Can you work these out from the drawing? Everything is in mm from the part's minimum corner. A direction names the side the tool comes from. Give positions to 0.01 mm unless a question says otherwise; leave off trailing zeros. Order: outer loops, then holes, each group sorted by start corner. A loop starts at its lowest first (then second) coordinate and runs counter-clockwise, first axis right, second up. Notation, with made-up numbers: M -30.5,-11.75 L -2.5,-11.75 A15 ccw -2.5,0.25 Z; hole C 42.25,6.5 d9. An arc over 180 degrees is marked long. Use a Markdown table: item, result. Add a question column.
Item 1: For the marked faces 1, 2 and 3, which set-ups out of +Z, -Z, +X, -X, +Y, -Y let a thin tool reach every point of the face, with its end or its side?
Item 2: I'm going to push flat-ended pins straight in: pin 1 Ø1 at (x, y) = (132, 4.5) entering from -Z; pin 2 Ø1 at (x, y) = (46, 5.5) entering from +Z; pin 3 Ø8 at (x, z) = (49.5, 20) entering from +Y (1 decimal). Where does each tip first touch, or does it pass through?
Item 3: Suppose I cut it at A-A on y = 4.5. Write out the boundary of the cut face in (x, z) (1 decimal).
Item 4: If I drill on L1, parallel to Y at x = 115.5, z = 83.5 (1 decimal); L2, parallel to Z at x = 42, y = 4.75, over which ranges is the centre line in solid material (lowest first)? Write a range as from..to.
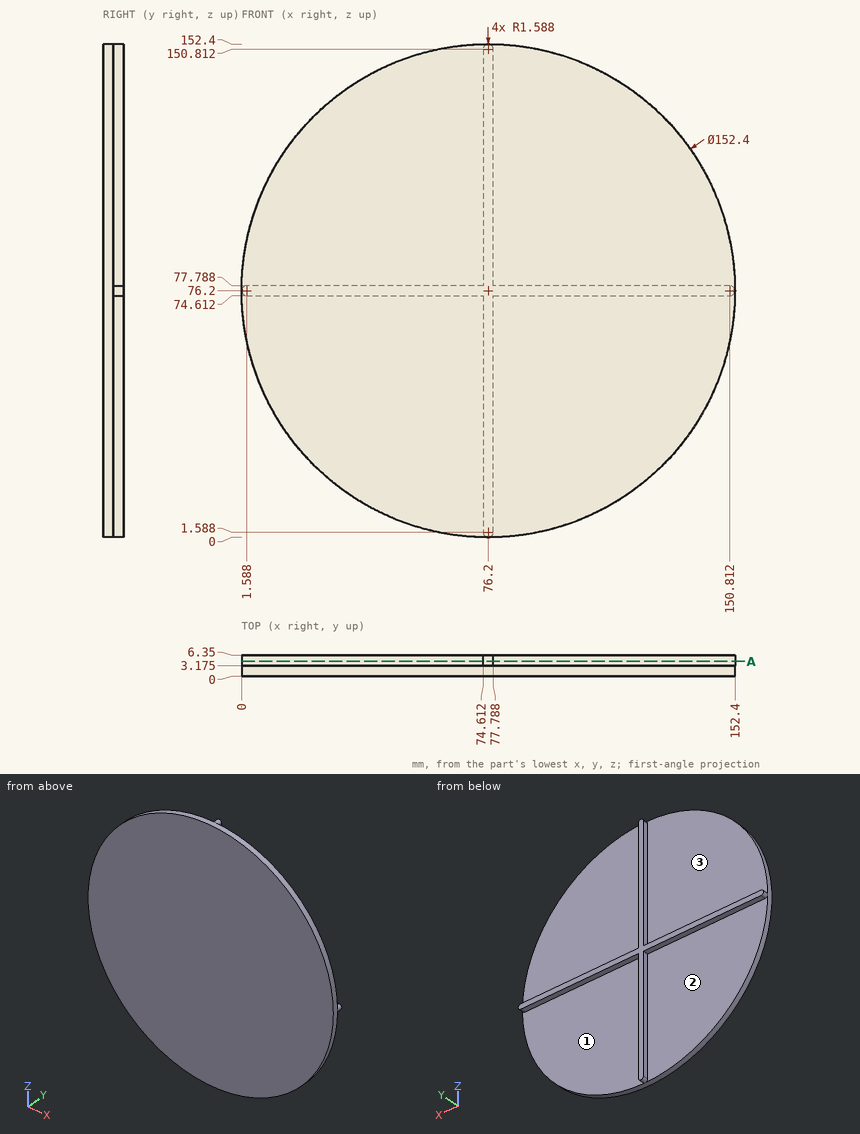
Findings below:
| question | item | result |
|---|---|---|
| 1 | face 1 | -Z, +X, +Y |
| 1 | face 2 | -Z, -X, +Y |
| 1 | face 3 | +Z, -X, +Y |
| 2 | pin 1 | stops at z = 74.61 |
| 2 | pin 2 | stops at z = 77.79 |
| 2 | pin 3 | stops at y = 3.2 |
| 3 | outline | M 1.6,74.6 L 74.6,74.6 L 74.6,1.6 A1.6 ccw 77.8,1.6 L 77.8,74.6 L 150.8,74.6 A1.6 ccw 150.8,77.8 L 77.8,77.8 L 77.8,150.8 A1.6 ccw 74.6,150.8 L 74.6,77.8 L 1.6,77.8 A1.6 ccw Z |
| 4 | L1 | y = 0..3.2 |
| 4 | L2 | z = 74.61..77.79 |
